Input: part model. Units: mm. Frame: model coordinates. Face numbers are marked on the shaded views. Coordinates: 2 decimals unless noted, no trailing zeros. Loops run counter-clockwise (first coordinate to the right, second up) from the corner with the lowest first, then second, coordinate; pieces in that order, holes last. Notation, with made-up numbers: (-2.5, -34.75) - (42.5, -34.75) arc R30 cw to (42.5, -3.75) - close; hole circle Ø5 at (-21.5, 36.25). An arc over 180 degrees is marked (long way). Write item = value, one per line. Start each with the question number.
from build123d import *

# Parameters (mm, degrees)
SKETCH_W     = 28
SKETCH_H     = 26
SKETCH_R     = 8
PAD_DEPTH    = 5
SKETCH001_R  = 2
POCKET_DEPTH = 26.001


with BuildPart() as part:
    # Sketch → Pad (new body)
    with BuildSketch(Plane.XY):
        Rectangle(SKETCH_W, SKETCH_H)
        Circle(SKETCH_R, mode=Mode.SUBTRACT)
    extrude(amount=PAD_DEPTH)

    # Sketch001 (on Face3 of Pad) → Pocket (cut, through all)
    with BuildSketch(Plane.XZ.offset(13)):
        with Locations((10, 2.5)):
            Circle(SKETCH001_R)
        with Locations((-10, 2.5)):
            Circle(SKETCH001_R)
    extrude(amount=-POCKET_DEPTH, mode=Mode.SUBTRACT)


solid = part.part
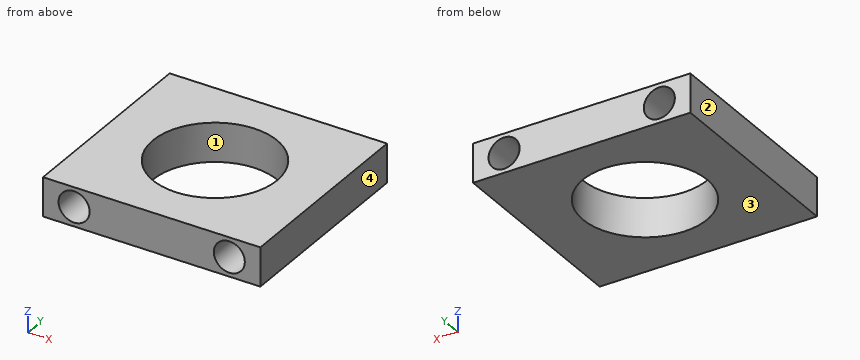
Item 1: Ray query, line 1 (Y direction, x = 0, z = 1.1); line 2 (Z direction, x = 10, y = -1); line 3 (X direction, y = -5, z = 2.4) (1 decimal). Return the intervals inside material, ascending.
Item 2: Cut plane B-B on y = 0. Return loops of the section in (x, z).
Item 3: Cut plane A-A on z = 2.5. Return loops of the section in (x, y).
Item 4: Cut plane C-C on x = 10. Return loops of the section in (y, z), plus the area to 3 significant figures.
Item 5: Cut plane D-D on y = -9.25. Return loops of the section in (x, z), plus the area to 3 significant figures.
Item 6: Pin query (flat end, axial travel): pin 1 (3 mm diameter, centred on x = 6, y = -9.5, fed in from -Z). Return the tip coordinate at first contact, or that it passes through.
Item 7: Pull-direction query (X, two-part tool) for the marked faces 1, 2, 3 and 4; classes: pulls with the +X half, pulls with the -X half, needs draft (parallel to the pull), parting line crosses it, or undercut.
Recorded:
q1.line_1 = -13 to -8, 8 to 13
q1.line_2 = 0 to 0.5, 4.5 to 5
q1.line_3 = -14 to -12, -8 to -6.2, 6.2 to 8, 12 to 14
q2.outline = (-14, 0) - (-8, 0) - (-8, 5) - (-14, 5) - close; (8, 0) - (14, 0) - (14, 5) - (8, 5) - close; hole circle Ø4 at (-10, 2.5); hole circle Ø4 at (10, 2.5)
q3.outline = (-14, -13) - (-12, -13) - (-12, 13) - (-14, 13) - close; (-8, -13) - (8, -13) - (8, 13) - (-8, 13) - close; (12, -13) - (14, -13) - (14, 13) - (12, 13) - close; hole circle Ø16 at (0, 0)
q4.outline = (-13, 0) - (13, 0) - (13, 0.5) - (-13, 0.5) - close; (-13, 4.5) - (13, 4.5) - (13, 5) - (-13, 5) - close
q4.area = 26.0 mm²
q5.outline = (-14, 0) - (14, 0) - (14, 5) - (-14, 5) - close; hole circle Ø4 at (-10, 2.5); hole circle Ø4 at (10, 2.5)
q5.area = 115 mm²
q6.pin_1 = 0
q7.face_1 = undercut
q7.face_2 = pulls with the -X half
q7.face_3 = needs draft
q7.face_4 = pulls with the +X half
